Could you check a few things on this model? Use its own coordinates, in mm. Face numbers are marked on the shaded views. A direction names the side the tool comes from. Coordinates: 2 decimals unless noted, no trailing zeros. Write item = value, one per line.
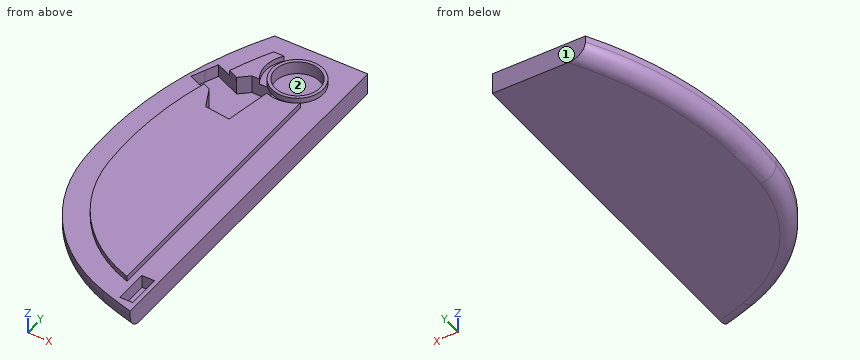
```python
from build123d import *

# Parameters (mm, degrees)
BOSS_EXTRUDE1_DEPTH = 10
FILLET1_R           = 7
CUT_EXTRUDE5_DEPTH  = 6
BOSS_EXTRUDE2_DEPTH = 2.5
SKETCH10_R          = 12
BOSS_EXTRUDE3_DEPTH = 2.5
SKETCH11_R          = 10.5
CUT_EXTRUDE6_DEPTH  = 6
SKETCH12_W          = 6
SKETCH12_H          = 16
CUT_EXTRUDE7_DEPTH  = 6


with BuildPart() as part:
    # Sketch1 → Boss-Extrude1 (new body)
    with BuildSketch(Plane.XY):
        with BuildLine():
            Line((0, 0), (-43.45, 0))
            ThreePointArc((-43.45, 0), (-62.674676093, -50.388720896), (-66.045303679, -104.214831977))
            ThreePointArc((-66.045303679, -104.214831977), (-50.462862729, -143.891349815), (-15.893438709, -168.83114646))
            ThreePointArc((-15.893438709, -168.83114646), (-7.994010798, -171.448872708), (0, -173.76171585))
            Line((0, -173.76171585), (0, 0))
        make_face()
    extrude(amount=BOSS_EXTRUDE1_DEPTH)

    # Fillet1
    fillet1_edges = [part.edges().sort_by_distance(p)[0] for p in [
        (-7.994010798, -171.448872708, 0),
        (-50.462862729, -143.891349815, 0),
        (-62.674676093, -50.388720896, 0),
    ]]
    fillet(fillet1_edges, radius=FILLET1_R)

    # Sketch7 → Cut-Extrude5 (cut)
    with BuildSketch(Plane.XY.offset(10)):
        Polygon((-55.192518946, -32.743925992), (-52.550619838, -26.805039808), (-40.67284747, -32.088838025), (-36.166399237, -28.159530493), (-24.434809325, -28.159530493), (-29.358040317, -55.413615039), (-41.316202905, -53.845312659), (-45.956645687, -43.966610392), (-57.834418054, -38.682812175), align=None)
    extrude(amount=-CUT_EXTRUDE5_DEPTH, mode=Mode.SUBTRACT)

    # Sketch9 → Boss-Extrude2 (add)
    with BuildSketch(Plane.XY.offset(10)):
        with BuildLine():
            Line((-11, -158.888662803), (-11, -32))
            ThreePointArc((-11, -32), (-17.986369061, -34.864228552), (-25.482975715, -33.961983287))
            Line((-25.482975715, -33.961983287), (-29.358040317, -55.413615039))
            Line((-29.358040317, -55.413615039), (-41.316202905, -53.845312659))
            Line((-41.316202905, -53.845312659), (-45.956645687, -43.966610392))
            Line((-45.956645687, -43.966610392), (-49.358199776, -42.453437309))
            ThreePointArc((-49.358199776, -42.453437309), (-55.003200537, -72.586352384), (-55.088286823, -103.243347748))
            ThreePointArc((-55.088286823, -103.243347748), (-41.773132254, -137.146827277), (-12.233650883, -158.457817531))
            ThreePointArc((-12.233650883, -158.457817531), (-11.617167152, -158.674218597), (-11, -158.888662803))
        make_face()
        with BuildLine():
            Line((-32, -11), (-36.901831421, -11))
            ThreePointArc((-36.901831421, -11), (-41.398196048, -20.383917403), (-45.30604713, -30.027770398))
            Line((-45.30604713, -30.027770398), (-40.67284747, -32.088838025))
            Line((-40.67284747, -32.088838025), (-36.166399237, -28.159530493))
            Line((-36.166399237, -28.159530493), (-32.586582623, -28.159530493))
            ThreePointArc((-32.586582623, -28.159530493), (-34.991243543, -19.487538254), (-32, -11))
        make_face()
    extrude(amount=BOSS_EXTRUDE2_DEPTH)

    # Sketch10 → Boss-Extrude3 (add)
    with BuildSketch(Plane.XY.offset(10)):
        with Locations((-20, -20)):
            Circle(SKETCH10_R)
    extrude(amount=BOSS_EXTRUDE3_DEPTH)

    # Sketch11 → Cut-Extrude6 (cut)
    with BuildSketch(Plane.XY.offset(12.5)):
        with Locations((-20, -20)):
            Circle(SKETCH11_R)
    extrude(amount=-CUT_EXTRUDE6_DEPTH, mode=Mode.SUBTRACT)

    # Sketch12 → Cut-Extrude7 (cut)
    with BuildSketch(Plane.XY.offset(10)):
        with Locations((-5, -160.76171585)):
            Rectangle(SKETCH12_W, SKETCH12_H)
    extrude(amount=-CUT_EXTRUDE7_DEPTH, mode=Mode.SUBTRACT)


solid = part.part
```
Item 1: For the marked faces 1 and 2, which set-ups out of +Z, -Z, +X, -X, +Y, -Y let a thin tool reach every point of the face, with its end or its side?
Numbers:
face_1 = +Z, -Z, +X, -X, +Y
face_2 = +Z
Item 2: I'm going to push flat-ended pins straight in: P1, Ø3, axis at x = -4.5, z = 6.5, coming from the +Y side; P2, Ø8, axis at x = -55, y = -23, coming from the +Z side; P3, Ø1.2, axis at x = -33.5, z = 11, coming from the +Y side; P4, Ø6, axis at x = -46, y = -145, coming from the -Z side. Where does each tip first touch, or does it pass through?
Numbers:
P1 = 0
P2 = 10
P3 = -11
P4 = 0.11
Item 3: If I drill on line 1 along Y through (x, z) = (-20, 10.2); line 2 along Z through (x, y) = (-9.5, -121.5); line 3 along Y through (x, z) = (-39, 4.5), over which ranges is the centre line in solid material (lowest first)?
Numbers:
line_1 = -155.13 to -35, -32 to -30.5, -9.5 to -8
line_2 = 0 to 10
line_3 = -155.13 to -54.15, -30.63 to 0
